Geometry check sheet. Reference: the model listing, model coordinates, mm. A direction names the side the tool comes from. Give positions to 0.01 mm unless a question says otherwise; leave off trailing zeros. Loops run counter-clockwise (first coordinate to the right, second up) from the corner with the lowest first, then second, coordinate; pieces in that order, holes last. Notation, with made-up numbers: (49, 22.5) -> (88, 22.5) arc R24 ccw to (88, 34.5) -> close; hole circle Ø8 at (4, 67). An arc over 180 degrees is marked (long way). One line per item, written item: value. Start each with the question number.
(1) Sectioned sample at B-B, the plane y = -2. Record the cut outline in (x, z).
(2) Sectioned sample at A-A, the plane z = 10.5. Record the cut outline in (x, y).
(3) Scan lines: line 1 along X through (y, z) = (9.5, -14); line 2 along Z through (x, y) = (-2, -1.6); line 3 along Y through (x, z) = (0.25, 8). Record each from-to range of solid material in increasing order. Write a range as from..to.
(4) Sectioned sample at D-D, the plane z = 4. Record the cut outline in (x, y).
(5) Tool access check on faces 1 (the face through (0, 0, 8)), 2 (the face through (-14, 0, -3)), 3 (the face through (10.308, 5.341, -13.035)). Record the directions out of +Z, -Z, +X, -X, +Y, -Y that give a thin tool (end or side, any length) a straight path to the whole face; none if there is none.
(6) Draft check along Z on faces 4 (the face through (0, -2, 15.5)), 5 (the face through (-10.15, 4.067, -8.096)), 6 (the face through (14, 0, -3)). Enter one of: pulls with the +Z half, pulls with the -Z half, needs draft (parallel to the pull), parting line crosses it, or undercut.
(7) Gauge pin test, flat ends, axial feed: pin 1 Ø5 at (x, z) = (-2, 10.5) entering from +Y; pin 2 Ø4 at (x, y) = (-8.5, 11.5) entering from +Z; pin 3 Ø4.5 at (y, z) = (8, -6.5) entering from -X. Record the tip position at first contact, or that the pin passes through.
from build123d import *

# Parameters (mm, degrees)
SKETCH_W        = 28
SKETCH_H        = 31
PAD_DEPTH       = 5
PAD001_DEPTH    = 28
SKETCH003_W     = 10
SKETCH003_H     = 15.030744
POCKET001_DEPTH = 15.586957
SKETCH005_R     = 3
POCKET_DEPTH    = 10.5
SKETCH006_R     = 1.75
POCKET003_DEPTH = 15.586957
SKETCH007_R     = 2
POCKET004_DEPTH = 5


with BuildPart() as part:
    # Sketch → Pad (new body)
    with BuildSketch(Plane.XZ):
        Rectangle(SKETCH_W, SKETCH_H)
    extrude(amount=PAD_DEPTH)

    # Sketch002 → Pad001 (join)
    with BuildSketch(Plane(origin=(14, 0, 0), x_dir=(0, 0, 1), z_dir=(1, 0, 0))):
        Polygon((-15.5, 0), (-0.028702, 0), (-15.5, -14.844726), align=None)
    extrude(amount=-PAD001_DEPTH)

    # Sketch003 (on DatumPlane) → Pocket001 (cut, through all)
    with BuildSketch(Plane(origin=(0, -0.014339, -0.013758), x_dir=(1, 0, 0), z_dir=(0, 0.020664, 0.999786))):
        with Locations((0, 7.659873)):
            Rectangle(SKETCH003_W, SKETCH003_H)
    extrude(amount=-POCKET001_DEPTH, mode=Mode.SUBTRACT)

    # Sketch005 (on DatumPlane) → Pocket (cut)
    with BuildSketch(Plane(origin=(0, -0.014339, -0.013758), x_dir=(1, 0, 0), z_dir=(0, 0.020664, 0.999786))):
        with Locations((-9.5, 7.175894)):
            Circle(SKETCH005_R)
        with Locations((9.5, 7.175894)):
            Circle(SKETCH005_R)
    extrude(amount=-POCKET_DEPTH, mode=Mode.SUBTRACT)

    # Sketch006 (on DatumPlane) → Pocket003 (cut, through all)
    with BuildSketch(Plane(origin=(0, -0.014339, -0.013758), x_dir=(1, 0, 0), z_dir=(0, 0.020664, 0.999786))):
        with Locations((-9.5, 7.175894)):
            Circle(SKETCH006_R)
        with Locations((9.5, 7.175894)):
            Circle(SKETCH006_R)
    extrude(amount=-POCKET003_DEPTH, mode=Mode.SUBTRACT)

    # Sketch007 (on DatumPlane) → Pocket004 (cut)
    with BuildSketch(Plane.XZ.offset(5)):
        with Locations((-1.65, -9.5)):
            Circle(SKETCH007_R)
        with Locations((-2, 10.5)):
            Circle(SKETCH007_R)
    extrude(amount=-POCKET004_DEPTH, mode=Mode.SUBTRACT)


solid = part.part
Calculated:
1. outline: (-14, -15.5) -> (14, -15.5) -> (14, 15.5) -> (-14, 15.5) -> close; hole circle Ø4 at (-2, 10.5); hole circle Ø4 at (-1.65, -9.5)
2. outline: (-14, -5) -> (-4, -5) -> (-4, 0) -> (-14, 0) -> close; (0, -5) -> (14, -5) -> (14, 0) -> (0, 0) -> close
3. line 1: x = -14..-5, 5..14
3. line 2: z = -15.5..-11.47, -7.53..8.5, 12.5..15.5
3. line 3: y = -5..0
4. outline: (-14, -5) -> (14, -5) -> (14, 0) -> (-14, 0) -> close
5. face 1: +Z, +X, -X, +Y
5. face 2: +Z, -Z, -X, +Y, -Y
5. face 3: none
6. face 4: pulls with the +Z half
6. face 5: undercut
6. face 6: needs draft
7. pin 1: stops at y = 0
7. pin 2: stops at z = -9.99
7. pin 3: stops at x = -14
